from build123d import *

# Parameters (mm, degrees)
SKETCH_1_R          = 8
EXTRUDE_1_DEPTH     = 70
SKETCH_6_R          = 1.5
CUT_EXTRUDE_1_DEPTH = 71
FILLET_1_R          = 0.3


with BuildPart() as part:
    # 草图1 → 凸台-拉伸1 (new body)
    with BuildSketch(Plane.XY):
        Circle(SKETCH_1_R)
    extrude(amount=-EXTRUDE_1_DEPTH)

    # 草图6 → 切除-拉伸1 (cut, through all)
    with BuildSketch(Plane.XY):
        Circle(SKETCH_6_R)
    extrude(amount=-CUT_EXTRUDE_1_DEPTH, mode=Mode.SUBTRACT)

    # 圆角1
    fillet_1_edges = [part.edges().sort_by_distance(p)[0] for p in [
        (-1.5, 0, -70),
        (-1.5, 0, 0),
    ]]
    fillet(fillet_1_edges, radius=FILLET_1_R)


solid = part.part
Work out the finished part from the listing and answer in its coordinate system (mm). Round coordinates to 2 decimals unless told otherwise and drop trailing zeros. Write each loop counter-clockwise with the first axis right and the second up, starting at its lowest first coordinate (ties: lowest second). Pieces come first, ordered by that corner, then holes. Notation, with made-up numbers: M -1,24.5 L 38,24.5 A32 cw 38,57.5 Z; hole C -27.75,46.5 d1. An arc over 180 degrees is marked long. Use a Markdown table: item, result.
1) Consider line 1 (Y direction, x = 0, z = -42.5); line 2 (Y direction, x = -1.25, z = -63); line 3 (X direction, y = 1, z = -15.5). Determine where each line is inside the solid, lowest interval first. Write a range as [from, to].
Taken from the geometry:
| item | result |
|---|---|
| line 1 | y = [-8, -1.5], [1.5, 8] |
| line 2 | y = [-7.9, -0.83], [0.83, 7.9] |
| line 3 | x = [-7.94, -1.12], [1.12, 7.94] |
2) Determine the mould class of faces 1 (the face through (-1.73, -7.81, -34.51)), 2 (the face through (0, 2, 0)), 3 (the face through (-1.5, 0.07, -34.51)) for opening direction X: pulls with the +X half, pulls with the -X half, needs draft (parallel to the pull), parting line crosses it, or undercut.
Taken from the geometry:
| item | result |
|---|---|
| face 1 | parting line crosses it |
| face 2 | needs draft |
| face 3 | undercut |
3) The part is cut by section C-C on z = -58. Give the vertices of the cut face in (x, y), plus the area to 3 significant figures.
Taken from the geometry:
| item | result |
|---|---|
| outline | C 0,0 d16; hole C 0,0 d3 |
| area | 194 mm2 |
4) The part is cut by section D-D on x = 6.75. Give the vertices of the cut face in (y, z).
Taken from the geometry:
| item | result |
|---|---|
| outline | M -4.29,-70 L 4.29,-70 L 4.29,0 L -4.29,0 Z |
5) Flat-ended cylindrical pins translate along their axes: pin 1 (4 mm diameter, centred on x = 3.5, z = -42.5, fed in from -Y); pin 2 (2.5 mm diameter, centred on x = 0, y = 0, fed in from +Z); pin 3 (1.5 mm diameter, centred on x = 1, z = -45, fed in from -Y); pin 4 (1.5 mm diameter, centred on y = -4.5, z = -35.5, fed in from -X). Find the tip coordinate at first contact, or state that the pin passes through.
Taken from the geometry:
| item | result |
|---|---|
| pin 1 | stops at y = -7.86 |
| pin 2 | passes through |
| pin 3 | stops at y = -8 |
| pin 4 | stops at x = -7.07 |
6) The part is cut by section A-A on y = 0. Give the vertices of the cut face in (x, z), plus the area to 3 significant figures.
Taken from the geometry:
| item | result |
|---|---|
| outline | M -8,-70 L -1.8,-70 A0.3 ccw -1.5,-69.7 L -1.5,-0.3 A0.3 ccw -1.8,0 L -8,0 Z; M 1.5,-69.7 A0.3 ccw 1.8,-70 L 8,-70 L 8,0 L 1.8,0 A0.3 ccw 1.5,-0.3 Z |
| area | 910 mm2 |
